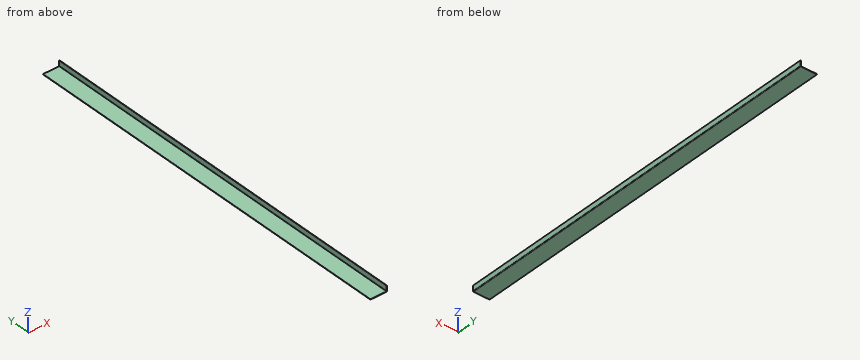
from build123d import *

# Parameters (mm, degrees)
SZKIC1_W                           = 95
SZKIC1_H                           = 2270
ODGI_CIE_BAZOWE1_DEPTH             = 2
ODGI_CIE_KRAW_DZI1_STRIP_W         = 9.4732
ODGI_CIE_KRAW_DZI1_STRIP_H         = 2
ODGI_CIE_KRAW_DZI1_STRIP_CUT_DEPTH = 2270
ODGI_CIE_KRAW_DZI1_DEPTH           = 2270


# Sheet-metal steps are written as plain solids
with BuildPart() as part:
    # Szkic1 → Odgięcie bazowe1 (new body)
    with BuildSketch(Plane.XY):
        with Locations((47.5, 1135)):
            Rectangle(SZKIC1_W, SZKIC1_H)
    extrude(amount=-ODGI_CIE_BAZOWE1_DEPTH)

    # Odgięcie krawędzi1 strip (across the edge) → Odgięcie krawędzi1 strip cut (cut)
    with BuildSketch(Plane(origin=(95, 0, 0), x_dir=(-1, 0, 0), z_dir=(0, 1, 0))):
        with Locations((-4, -1)):
            Rectangle(ODGI_CIE_KRAW_DZI1_STRIP_W, ODGI_CIE_KRAW_DZI1_STRIP_H)
    extrude(amount=ODGI_CIE_KRAW_DZI1_STRIP_CUT_DEPTH, mode=Mode.SUBTRACT)

    # Odgięcie krawędzi1 section (across the edge) → Odgięcie krawędzi1 (add)
    with BuildSketch(Plane(origin=(95, 0, 0), x_dir=(-1, 0, 0), z_dir=(0, 1, 0))):
        with BuildLine():
            Line((-2, 0.7366), (-2, 30.74))
            Line((-2, 30.74), (0, 30.74))
            Line((0, 30.74), (0, 0.7366))
            ThreePointArc((0, 0.7366), (0.215745145, 0.215745145), (0.7366, 0))
            Line((0.7366, 0), (0.7366, -2))
            ThreePointArc((0.7366, -2), (-1.198468417, -1.198468417), (-2, 0.7366))
        make_face()
    extrude(amount=ODGI_CIE_KRAW_DZI1_DEPTH)


solid = part.part
Verification items for the finished model (mm, model axes). Give positions to 0.01 mm unless a question says otherwise; leave off trailing zeros. Write each loop counter-clockwise with the first axis right and the second up, starting at its lowest first coordinate (ties: lowest second). Pieces come first, ordered by that corner, then holes. Notation, with made-up numbers: M -40,-13.5 L -17,-13.5 A10 cw -17,-7.5 Z; hole C 26,-31 d2. An arc over 180 degrees is marked long. Use CSV: the item, a comma, the result in double quotes.
1) Cross-section at A-A (y = 951.5). Enter the section's corners in (x, z), plus the area to 3 significant figures.
Final values:
outline,"M 0,-2 L 94.26,-2 A2.74 ccw 97,0.74 L 97,30.74 L 95,30.74 L 95,0.74 A0.74 cw 94.26,0 L 0,0 Z"
area,"254 mm²"
2) Cross-section at B-B (z = 16). Enter the section's corners in (x, y), plus the area to 3 significant figures.
Final values:
outline,"M 95,0 L 97,0 L 97,2270 L 95,2270 Z"
area,"4,540 mm²"
3) Go/stop test with a flat-tipped pin: pin 1 Ø1.5 at (y, z) = (285, 2) entering from -X. Record where the tip stops, or that it passes through.
Final values:
pin 1,"x = 95"
4) Cross-section at C-C (x = 54.5). Enter the section's corners in (y, z), plus the area to 3 significant figures.
Final values:
outline,"M 0,-2 L 2270,-2 L 2270,0 L 0,0 Z"
area,"4,540 mm²"
5) Material ranges on line 1 along X through (y, z) = (1995, 4.5); line 2 along Z through (x, y) = (33.5, 1106.5), recorded low to high.
Final values:
line 1,"95 to 97"
line 2,"-2 to 0"
